from build123d import *

# Parameters (mm, degrees)
SKETCH1_W           = 100
SKETCH1_H           = 100
BOSS_EXTRUDE1_DEPTH = 500
SKETCH2_W           = 168
SKETCH2_H           = 20
BOSS_EXTRUDE2_DEPTH = 400
BOSS_EXTRUDE3_DEPTH = 400


with BuildPart() as part:
    # Sketch1 → Boss-Extrude1 (new body)
    with BuildSketch(Plane.XY):
        with Locations((50, 50)):
            Rectangle(SKETCH1_W, SKETCH1_H)
    extrude(amount=BOSS_EXTRUDE1_DEPTH)

    # Sketch2 → Boss-Extrude2 (add)
    with BuildSketch(Plane.XY.offset(500)):
        with Locations((50, 10)):
            Rectangle(SKETCH2_W, SKETCH2_H)
    extrude(amount=BOSS_EXTRUDE2_DEPTH)

    # Sketch3 → Boss-Extrude3 (add)
    with BuildSketch(Plane.XY.offset(900)):
        Polygon((134, 0), (291.868360292, -57.459384079), (298.296236389, -39.798939648), (134, 20), align=None)
        Polygon((-198.296236389, -39.798939648), (-34, 20), (-34, 0), (-191.868360292, -57.459384079), align=None)
    extrude(amount=-BOSS_EXTRUDE3_DEPTH)


solid = part.part
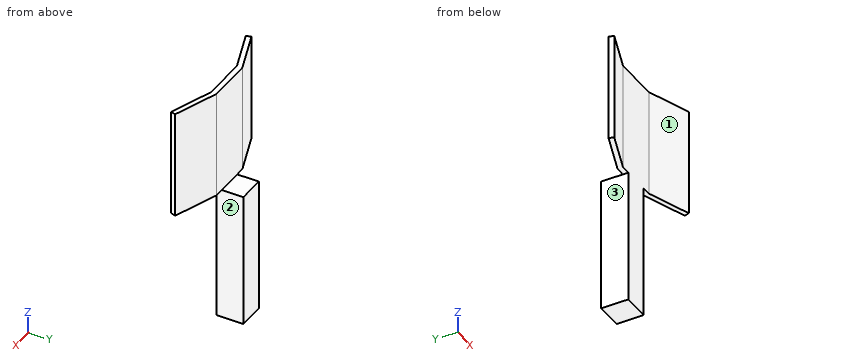
Can you work these out from the model? Positions are in its coordinate system, mm. Face numbers are marked on the shaded views. A direction names the side the tool comes from. Coordinates: 2 decimals unless noted, no trailing zeros. Write each loop counter-clockwise with the first axis right and the second up, starting at its lowest first coordinate (ties: lowest second). Pieces come first, ordered by that corner, then holes.
Q1. Imagine slicing it at A-A, the plane y = -23. List the corners of the cut face in (x, z) for me.
Results found:
outline: (-152.14, 500) - (-97.19, 500) - (-97.19, 900) - (-152.14, 900) - close; (197.19, 500) - (252.14, 500) - (252.14, 900) - (197.19, 900) - close
Q2. Please list where these lines run through material, in increasing order: L1, parallel to Z at x = 251.5, y = -37; L2, parallel to X at y = 48, z = 310.5.
Results found:
L1: z = 500 to 900
L2: x = 0 to 100
Q3. For P1, Ø4, axis at x = 72, z = 254, coming from the -Y side; P2, Ø8, axis at y = -6.5, z = 301.5, coming from the -X side; P3, Ø10, axis at x = 79.5, z = 741, coming from the +Y side; P4, Ø24, axis at x = 39.5, y = 56, coming from the +Z side, each with a flat end and sliding along its axis, tell me the tip position at first contact or that it passes through.
Results found:
P1: stops at y = 0
P2: passes through
P3: stops at y = 20
P4: stops at z = 500
Q4. Imagine slicing it at D-D, the plane y = 30. List the corners of the cut face in (x, z) for me, plus the area to 3 significant figures.
Results found:
outline: (0, 0) - (100, 0) - (100, 500) - (0, 500) - close
area: 50,000 mm2
Q5. Imagine slicing it at C-C, the plane x = 67.5. List the corners of the cut face in (y, z) for me.
Results found:
outline: (0, 0) - (100, 0) - (100, 500) - (20, 500) - (20, 900) - (0, 900) - close
Q6. Which directions (+Z, -Z, +X, -X, +Y, -Y) give clear straight access to the entire face, cutting with the end or side of a thin tool? Please do the marked faces 1, 2 and 3.
Results found:
face 1: +Z, -Z, -Y
face 2: -Z, +X, +Y, -Y
face 3: -Z, -X, +Y, -Y
Q7. Imagine slicing it at B-B, the plane z = 545.5. List the corners of the cut face in (x, y) for me, plus the area to 3 significant figures.
Results found:
outline: (-198.3, -39.8) - (-191.87, -57.46) - (-34, 0) - (134, 0) - (291.87, -57.46) - (298.3, -39.8) - (134, 20) - (-34, 20) - close
area: 9,800 mm2
